```python
from build123d import *

# Parameters (mm, degrees)
BOSS_EXTRUDE2_DEPTH = 4.5
SKETCH3_R           = 1.3
CUT_EXTRUDE1_DEPTH  = 10.5
SKETCH6_W           = 2.938556516
SKETCH6_H           = 1.727001967
BOSS_EXTRUDE5_DEPTH = 17


with BuildPart() as part:
    # Sketch1 → Boss-Extrude2 (new body)
    with BuildSketch(Plane(origin=(0, 0, 0), x_dir=(0, 0, -1), z_dir=(1, 0, 0))):
        with BuildLine():
            Line((1.55613054, -9.91539795), (3.9164982, -9.916319844))
            Line((3.9164982, -9.916319844), (3.9164982, -4.895563354))
            ThreePointArc((3.9164982, -4.895563354), (4.059992057, -1.782444065), (4.214804462, -4.895021022))
            Line((4.214804462, -4.895021022), (4.214804462, -9.916436354))
            Line((4.214804462, -9.916436354), (6.579674081, -9.917360006))
            Line((6.579674081, -9.917360006), (6.579674081, -0.928463249))
            Line((6.579674081, -0.928463249), (1.55613054, -0.928463249))
            Line((1.55613054, -0.928463249), (1.55613054, -9.91539795))
        make_face()
    extrude(amount=BOSS_EXTRUDE2_DEPTH)

    # Sketch3 → Cut-Extrude1 (cut)
    with BuildSketch(Plane.XY.offset(-1.55613054)):
        with Locations((2.256029543, -7.121731935)):
            Circle(SKETCH3_R)
    extrude(amount=-CUT_EXTRUDE1_DEPTH, mode=Mode.SUBTRACT)

    # Sketch6 → Boss-Extrude5 (add)
    with BuildSketch(Plane(origin=(0, -0.928463249, 0), x_dir=(1, 0, 0), z_dir=(0, 1, 0))):
        with Locations((2.247156979, 4.067903294)):
            Rectangle(SKETCH6_W, SKETCH6_H)
    extrude(amount=BOSS_EXTRUDE5_DEPTH)


solid = part.part
```
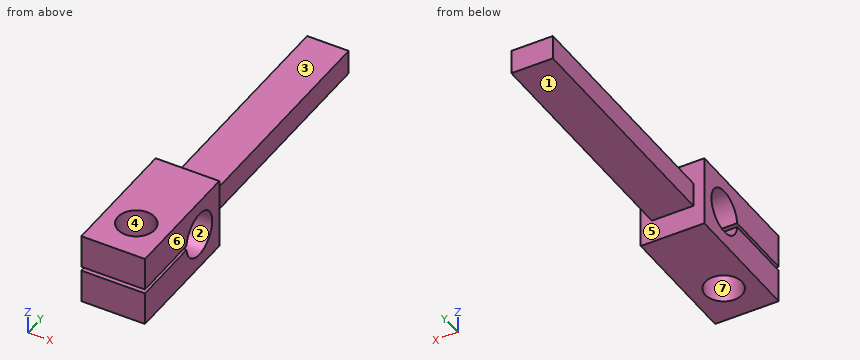
The listing builds one solid part. Answer for the finished solid, in the listing's coordinates (mm). Face numbers are marked on the shaded views. A direction names the side the tool comes from. Round coordinates to 2 decimals unless told otherwise and drop trailing zeros. Write each loop counter-clockwise with the first axis right and the second up, starting at its lowest first coordinate (ties: lowest second). Pieces come first, ordered by that corner, then holes. Notation, with made-up numbers: (-28.5, 10.25) -> (8.5, 10.25) arc R17 cw to (8.5, 35.25) -> close; hole circle Ø4 at (-8.75, 11.25). An arc over 180 degrees is marked (long way). Use CSV: the item, a comma, the result in double quotes. Start each with the question number.
(1) Consider L1, parallel to Z at x = 0.4, y = -5.75; L2, parallel to Y at x = 1.5, z = -2.7; L3, parallel to Z at x = 2.6, y = 1.25. Determine where each line is inside the solid, lowest interval first. Write a range as from..to.
(2) Section D-D on z = -5.85 is taken. Give the vertices of the cut face in (x, y).
(3) The mould has two halves that part along X. Classify the marked faces 4, 5, 6 and 7: released by +X, released by -X, zero draft, split by the parting line, or undercut.
(4) Section C-C on x = 0.3 is taken. Give the vertices of the cut face in (y, z).
(5) Each of these flat-tipped pins is pushed along its axis until it touches: pin 1 (2 mm diameter, centred on x = 2.26, y = -7.12, fed in from -Z); pin 2 (1.9 mm diameter, centred on y = 8, z = -4.5, fed in from +X); pin 3 (0.5 mm diameter, centred on y = 6, z = -4, fed in from -X); pin 4 (2.5 mm diameter, centred on x = 3, y = 7.5, fed in from -Z). Where does it stop, or does it pass through?
(6) Section A-A on x = 3.05 is taken. Give the vertices of the cut face in (y, z).
(7) Section B-B on y = -3.5 is taken. Give the vertices of the cut face in (x, z), then the cut area to 3 significant figures.
(8) Which of the six approach directions +Z, -Z, +X, -X, +Y, -Y give full straight-line access (tool end or side, diameter ignored) to the marked faces 1, 2 and 3?
A:
1,L1,"z = -6.58..-4.21, -3.92..-1.56"
1,L2,"y = -9.92..-8.18, -6.06..-4.1, -2.58..-0.93"
1,L3,"z = -4.93..-3.2"
2,outline,"(0, -9.92) -> (4.5, -9.92) -> (4.5, -0.93) -> (0, -0.93) -> close; hole circle Ø2.6 at (2.26, -7.12)"
3,face 4,"undercut"
3,face 5,"zero draft"
3,face 6,"released by +X"
3,face 7,"undercut"
4,outline,"(-9.92, -6.58) -> (-0.93, -6.58) -> (-0.93, -1.56) -> (-9.92, -1.56) -> (-9.92, -3.92) -> (-4.9, -3.92) arc R1.56 cw (long way) to (-4.9, -4.21) -> (-9.92, -4.21) -> close"
5,pin 1,"passes through"
5,pin 2,"stops at x = 3.72"
5,pin 3,"stops at x = 0.78"
5,pin 4,"stops at z = -4.93"
6,outline,"(-9.92, -6.58) -> (-8.15, -6.58) -> (-8.15, -4.21) -> (-9.92, -4.21) -> close; (-9.92, -3.92) -> (-8.15, -3.92) -> (-8.15, -1.56) -> (-9.92, -1.56) -> close; (-6.09, -6.58) -> (-0.93, -6.58) -> (-0.93, -4.93) -> (16.07, -4.93) -> (16.07, -3.2) -> (-0.93, -3.2) -> (-0.93, -1.56) -> (-6.09, -1.56) -> (-6.09, -3.92) -> (-4.9, -3.92) arc R1.56 cw (long way) to (-4.9, -4.21) -> (-6.09, -4.21) -> close"
7,outline,"(0, -6.58) -> (4.5, -6.58) -> (4.5, -5.61) -> (0, -5.61) -> close; (0, -2.51) -> (4.5, -2.51) -> (4.5, -1.56) -> (0, -1.56) -> close"
7,area,"8.64 mm²"
8,face 1,"-Z, +X, -X, +Y"
8,face 2,"+X, -X"
8,face 3,"+Z, +X, -X, +Y"
